from build123d import *

# Parameters (mm, degrees)
F1_DEPTH = 600
F2_W     = 760
F2_H     = 300
F3_DEPTH = 80
F4_W     = 150
F4_H     = 440
F5_DEPTH = 20
F6_SIZE  = 20
F7_R     = 15


with BuildPart() as f1:
    # F0 (on Front) → F1 (new body)
    with BuildSketch(Plane.XZ):
        Polygon((-220, 0), (0, 0), (0, 390), (-700, 390), (-700, 0), (-480, 0), (-425, 190), (-275, 190), align=None)
    extrude(amount=F1_DEPTH)

    # F2 (on face) → F3 (cut)
    with BuildSketch(Plane(origin=(0, 0, 0), x_dir=(1, 0, 0), z_dir=(0, 0, -1))):
        with Locations((-350, 300)):
            Rectangle(F2_W, F2_H)
    extrude(amount=-F3_DEPTH, mode=Mode.SUBTRACT)

    # F4 (on face) → F5 (cut)
    with BuildSketch(Plane(origin=(0, 0, 190), x_dir=(1, 0, 0), z_dir=(0, 0, -1))):
        with Locations((-350, 300)):
            Rectangle(F4_W, F4_H)
    extrude(amount=-F5_DEPTH, mode=Mode.SUBTRACT)

    # F6
    f6_edges = [f1.edges().sort_by_distance(p)[0] for p in [
        (-700, 0, 195),
        (-700, -300, 390),
        (-350, 0, 390),
        (0, -300, 390),
        (-350, -600, 390),
        (-700, -600, 195),
        (0, -600, 195),
        (0, 0, 195),
    ]]
    chamfer(f6_edges, length=F6_SIZE)

    # F7
    f7_edges = [f1.edges().sort_by_distance(p)[0] for p in [
        (-275, -520, 200),
        (-425, -520, 200),
        (-425, -80, 200),
        (-275, -80, 200),
    ]]
    fillet(f7_edges, radius=F7_R)


solid = f1.part
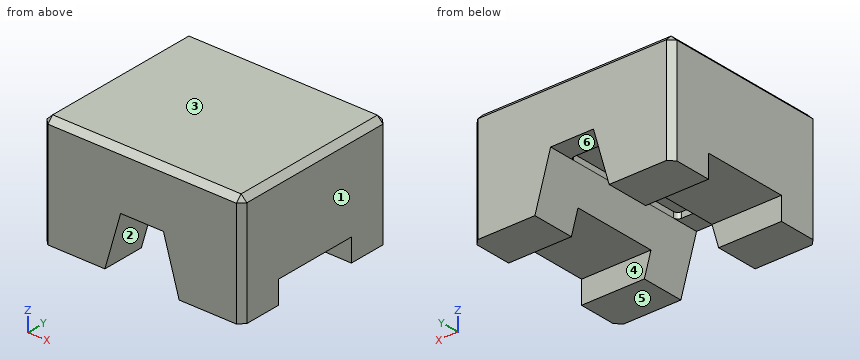
CAD build for the part. Positions are in the model's coordinates, mm. Face numbers are marked on the shaded views. A direction names the side the tool comes from. Round coordinates to 2 decimals unless told otherwise and drop trailing zeros. Loops run counter-clockwise (first coordinate to the right, second up) from the corner with the lowest first, then second, coordinate; pieces in that order, holes last. Notation, with made-up numbers: (9, 35) - (36, 35) arc R10 ccw to (36, 43) - close; hole circle Ø1 at (70.5, 2.5). An arc over 180 degrees is marked (long way). Put each result on its own line as item: value.
1. 3-axis set-ups, long thin cutter, end or side, ignore diameter. For the marked faces 4, 5 and 6: which of +Z, -Z, +X, -X, +Y, -Y reach the whole face in a straight line?
Geometry check:
face 4: -Z, +X, -X
face 5: -Z, +X, -X, +Y, -Y
face 6: -Z, +Y, -Y
2. Two-plate mould, pull along X, no slides. Class the marked faces 1, 2 and 3: released by +X, released by -X, zero draft, split by the parting line, or undercut.
Geometry check:
face 1: released by +X
face 2: undercut
face 3: zero draft
3. Wall check: line 1 (X direction, y = -422, z = 194.5); line 2 (Z direction, x = -374, y = -476); line 3 (Z direction, x = -86.5, y = -239). Give the ranges that are in metal, low to high.
Geometry check:
line 1: -700 to -425, -275 to 0
line 2: 210 to 390
line 3: 80 to 390
4. Pin check, flat tip, straight feed: P1, Ø5, axis at x = -486, y = -406, coming from the -Z side. Stop position of the tip, or through.
Geometry check:
P1: z = 80
5. Slice it at C-C on y = -181.5. List the corners of the cut face in (x, z), and give its area (3 significant figures).
Geometry check:
outline: (-700, 80) - (-456.84, 80) - (-425, 190) - (-425, 210) - (-275, 210) - (-275, 190) - (-243.16, 80) - (0, 80) - (0, 370) - (-20, 390) - (-680, 390) - (-700, 370) - close
area: 194,000 mm²
6. Slice it at D-D on y = -473. List the corners of the cut face in (x, z), and give its area (3 significant figures).
Geometry check:
outline: (-700, 0) - (-480, 0) - (-425, 190) - (-425, 210) - (-275, 210) - (-275, 190) - (-220, 0) - (0, 0) - (0, 370) - (-20, 390) - (-680, 390) - (-700, 370) - close
area: 231,000 mm²
7. Slice it at A-A on z = 92. List the corners of the cut face in (x, y), and give its area (3 significant figures).
Geometry check:
outline: (-700, -580) - (-680, -600) - (-453.37, -600) - (-453.37, 0) - (-680, 0) - (-700, -20) - close; (-246.63, -600) - (-20, -600) - (0, -580) - (0, -20) - (-20, 0) - (-246.63, 0) - close
area: 295,000 mm²
8. Slice it at B-B on x = -204. List the corners of the cut face in (y, z).
Geometry check:
outline: (-600, 0) - (-450, 0) - (-450, 80) - (-150, 80) - (-150, 0) - (0, 0) - (0, 370) - (-20, 390) - (-580, 390) - (-600, 370) - close
